Geometry check sheet. Reference: the model listing, model coordinates, mm. Face numbers are marked on the shaded views. A direction names the side the tool comes from. Coordinates: 2 decimals unless noted, no trailing zeros. Loops run counter-clockwise (first coordinate to the right, second up) from the corner with the lowest first, then second, coordinate; pieces in that order, holes last. Notation, with made-up numbers: (73, 30) - (101, 30) arc R29 cw to (101, 52) - close; hole circle Ø10 at (-3, -4.75). An arc over 180 degrees is marked (long way). Write each question's results on one line, items separated by ' | '. Start each with the question number.
(1) Access from +Z, -Z, +X, -X, +Y, -Y to the whole of each face (thin tool, end or side, straight path). Record for the marked faces 1, 2 and 3.
(2) Sectioned sample at A-A (z = 4.5). Enter the section's corners in (x, y), plus the area to 3 significant figures.
(3) Material ranges on probe 1 along Z at (x, y) = (-1.7, 36); probe 2 along X at (y, z) = (34.25, -1); probe 3 along X at (y, z) = (35.5, 15), recorded low to high.
(4) Go/stop test with a flat-tipped pin: pin 1 Ø1 at (y, z) = (34.5, 16.5) entering from +X. Record where the tip stops, or that it passes through.
Autodesk Inventor part; units mm, degrees
ref_plane "Work Plane1" through (0, 38.1, 0) normal (0, 1, 0) x (-1, 0, 0)
ref_plane "YZ Plane" through (0, 0, 0) normal (1, 0, 0) x (0, 1, 0)
ref_plane "XY Plane" through (0, 0, 0) normal (0, 0, 1) x (1, 0, 0)
sketch "Sketch6" plane through (0, 0, 0) normal (0, 1, 0) x (-1, 0, 0)
  line L0 (0, 0) -> (5.588, 0)
  line L1 (5.588, 0) -> (5.588, -6.35)
  line L2 (5.588, -6.35) -> (0, -6.35)
  line L3 (0, -6.35) -> (0, 0)
  arc A0 (0, -6.35) -> (5.588, -6.35) centre (2.794, -6.35) ccw
  dimension "d25" = 5.588
  dimension "d26" = 6.35
ref_plane "Work Plane1" through (0, 38.1, 0) normal (0, 1, 0) x (-1, 0, 0)
sketch "Sketch8" plane through (0, 38.1, 0) normal (0, 1, 0) x (-1, 0, 0)
  line L0 (4.3815, 0) -> (1.2065, 0)
  line L1 (1.2065, 0) -> (1.2065, -3.81)
  line L2 (1.2065, -3.81) -> (4.3815, -3.81)
  line L3 (4.3815, -3.81) -> (4.3815, 0)
  arc A0 (1.2065, -3.81) -> (4.3815, -3.81) centre (2.794, -3.81) ccw
  point P0 (0, 0)
  dimension "d27" = 3.175
  dimension "d28" = 3.81
  dimension "d49" = 1.2065
loft "Loft1" add profiles "Sketch6", "Sketch8"
sketch "Sketch9" plane through (-5.588, 0, 0) normal (0, 0, 1) x (1, 0, 0)
  line L0 (0, 0) -> (5.588, 0)
  line L1 (5.588, 0) -> (4.3815, 38.1)
  line L2 (1.2065, 38.1) -> (4.3815, 38.1)
  line L3 (0, 0) -> (1.2065, 38.1)
  line L4 (4.3815, 38.1) -> (5.588, 0)
  line L5 (4.5826, 31.75) -> (1.0054, 31.75)
  line L6 (0, 0) -> (1.2065, 38.1)
  dimension "d34" = 6.35
extrude "Extrusion5" add sketch "Sketch9" along normal blind 38.608 contours L3 L2 L1 L5
sketch "Sketch12" plane through (-2.794, 0, -6.35) normal (0, -1, 0) x (1, 0, 0)
  circle A0 centre (0, 1.9685) radius 1.27
  arc A1 (-2.794, 0) -> (2.794, 0) centre (0, 0) ccw
  line L0 (0, -2.794) -> (0, 1.9685)
  point P0 (2.794, 6.35)
  dimension "d44" = 2.54
  dimension "d46" = 4.7625
extrude "Extrusion8" cut sketch "Sketch12" against normal blind 10.16
sketch "Sketch13" plane through (-5.588, 0, 0) normal (0, 0, 1) x (1, 0, 0)
  line L0 (1.2065, 38.1) -> (4.3815, 38.1)
  line L1 (3.6195, 38.1) -> (1.9685, 38.1)
  line L2 (1.9685, 38.1) -> (1.9685, 31.75)
  line L3 (1.9685, 31.75) -> (3.6195, 31.75)
  line L4 (3.6195, 31.75) -> (3.6195, 38.1)
  line L5 (3.6195, 31.75) -> (4.5826, 31.75) construction
  line L6 (4.3815, 38.1) -> (5.588, 0) construction
  line L7 (1.9685, 31.75) -> (1.0054, 31.75) construction
  line L8 (0, 0) -> (1.2065, 38.1) construction
  line L9 (10.391, 31.75) -> (-0.9915, 31.75)
  line L10 (-0.9915, 31.75) -> (-0.9915, -4.8332)
  line L11 (-0.9915, -4.8332) -> (10.391, -4.8332)
  line L12 (10.391, -4.8332) -> (10.391, 31.75)
  line L13 (1.9685, 38.1) -> (1.2065, 38.1)
  line L14 (1.9685, 31.75) -> (1.0054, 31.75)
  line L15 (1.0054, 31.75) -> (1.2065, 38.1)
  line L16 (3.6195, 38.1) -> (4.3815, 38.1)
  line L17 (4.3815, 38.1) -> (4.5826, 31.75)
  line L18 (3.6195, 31.75) -> (4.5826, 31.75)
  dimension "d50" = 1.651
  dimension "d51" = 6.35
extrude "Extrusion11" cut sketch "Sketch13" against normal through all contours L0 L2 L9 L15 | L0 L17 L9 L4
extrude "Extrusion12" cut sketch "Sketch13" against normal through all contours L9 L3 L12 L11 L10
properties part number "RudderStabilizingFinBottom_Print2"
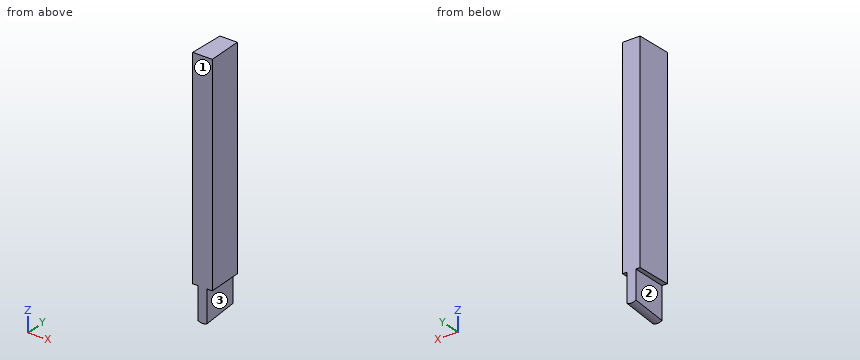
Outcome:
1) face 1: +Z, -Z, +X, -X, -Y | face 2: -Z, -X, +Y, -Y | face 3: -Z, +X, +Y, -Y
2) outline: (-4.58, 31.75) - (-1.01, 31.75) - (-1.21, 38.1) - (-4.38, 38.1) - close | area: 21.4 mm2
3) probe 1: z = 0 to 38.61 | probe 2: x = -3.62 to -1.97 | probe 3: x = -4.46 to -1.12
4) pin 1: stops at x = -1.08
